Check sheet for the modelled part. Datum: model origin and axes. Units: mm. Face numbers are marked on the shaded views. Give positions to 0.01 mm unless a question says otherwise; leave off trailing zeros. Order: outer loops, then holes, each group sorted by start corner. A loop starts at its lowest first (then second) coordinate and runs counter-clockwise, first axis right, second up. Notation, with made-up numbers: (28.25, -19) -> (38.25, -19) arc R21 cw to (38.25, 12) -> close; hole circle Ø10 at (47.25, -31). An arc over 180 degrees is marked (long way). Write each question's results on one line, items separated by ' | '.
from build123d import *

# Parameters (mm, degrees)
SKETCH006_W      = 50
SKETCH006_H      = 30
EXTRUDE006_DEPTH = 70
SKETCH007_W      = 50
SKETCH007_H      = 60
EXTRUDE007_DEPTH = 60
SKETCH005_W      = 50
SKETCH005_H      = 60
EXTRUDE005_DEPTH = 500


with BuildPart() as obj1:
    # Sketch006 (on Face6 of Extrude005) → Extrude006 (new body)
    with BuildSketch(Plane.XY.offset(630)):
        with Locations((570, 45)):
            Rectangle(SKETCH006_W, SKETCH006_H)
    extrude(amount=EXTRUDE006_DEPTH)


with BuildPart() as obj2:
    # Sketch007 (on Face6 of Extrude006) → Extrude007 (new body)
    with BuildSketch(Plane.XY.offset(700)):
        with Locations((570, 30)):
            Rectangle(SKETCH007_W, SKETCH007_H)
    extrude(amount=EXTRUDE007_DEPTH)


with BuildPart() as fusion:
    # Sketch005 (on Face14 of Extrude004) → Extrude005 (new body)
    with BuildSketch(Plane.XY.offset(130)):
        with Locations((570, 30)):
            Rectangle(SKETCH005_W, SKETCH005_H)
    extrude(amount=EXTRUDE005_DEPTH)

    # Fusion: union obj1, obj2
    add(obj1.part)
    add(obj2.part)


with BuildPart() as fusion_mirrored:
    # mirror: instance of Fusion
    add(fusion.part.mirror(Plane(origin=(1140, 300, 120), x_dir=(1, 0, 0), z_dir=(0, 1, 0))))


solid = fusion_mirrored.part
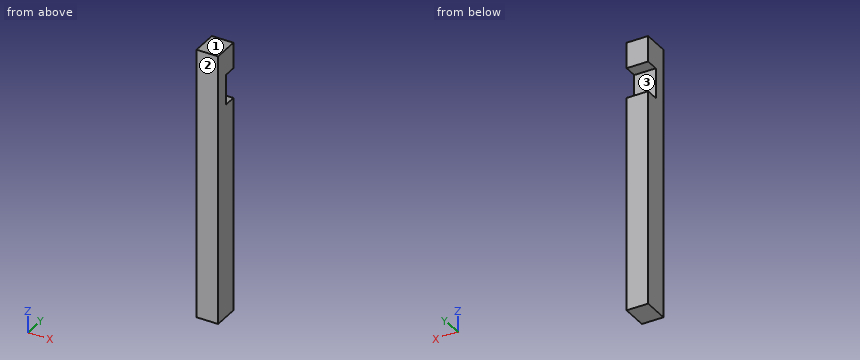
1. Material ranges on probe 1 along Z at (x, y) = (562, 592); probe 2 along Y at (x, z) = (556, 631), recorded low to high. Write a range as from..to.
Verdict:
probe 1: z = 130..630, 700..760 | probe 2: y = 540..570
2. Section check B-B on x = 561.5. Record the cut outline in (y, z).
Verdict:
outline: (540, 130) -> (600, 130) -> (600, 630) -> (570, 630) -> (570, 700) -> (600, 700) -> (600, 760) -> (540, 760) -> close
3. Section check A-A on y = 585.5. Record the cut outline in (x, z).
Verdict:
outline: (545, 130) -> (595, 130) -> (595, 630) -> (545, 630) -> close; (545, 700) -> (595, 700) -> (595, 760) -> (545, 760) -> close
4. Mould release check, pull along Z, two halves, no side actions. Record for the marked faces 1, 2 and 3: +Z half, -Z half, draft (parallel to the pull), parting line (faces both ways), or undercut.
Verdict:
face 1: +Z half | face 2: draft | face 3: undercut
